Work out the finished part from the listing and answer in its coordinate system (mm). A direction names the side the tool comes from. Round coordinates to 2 decimals unless told otherwise and drop trailing zeros. Loops run counter-clockwise (first coordinate to the right, second up) from the corner with the lowest first, then second, coordinate; pieces in that order, holes last.
```python
from build123d import *

# Parameters (mm, degrees)
F1_DEPTH = 1000


with BuildPart() as f1:
    # F0 (on Right) → F1 (new body)
    with BuildSketch(Plane.YZ):
        with BuildLine():
            Line((0, 73.95), (0, 0.5))
            ThreePointArc((0, 0.5), (0.146447, 0.146447), (0.5, 0))
            Line((0.5, 0), (1.1, 0))
            ThreePointArc((1.1, 0), (1.453553, 0.146447), (1.6, 0.5))
            Line((1.6, 0.5), (1.6, 76.2))
            Line((1.6, 76.2), (77.798804, 76.2))
            Line((77.798804, 76.2), (77.798804, 77.2))
            Line((77.798804, 77.2), (1.598804, 77.2))
            Line((1.598804, 77.2), (1.598804, 79.3))
            Line((1.598804, 79.3), (2.548804, 79.3))
            ThreePointArc((2.548804, 79.3), (2.696007, 79.118338), (2.919614, 79.05))
            Line((2.919614, 79.05), (3.348827, 79.05))
            ThreePointArc((3.348827, 79.05), (3.524228, 79.121858), (3.598797, 79.296124))
            Line((3.598797, 79.296124), (3.598857, 79.3))
            Line((3.598857, 79.3), (3.598857, 80.9))
            Line((3.598857, 80.9), (0, 80.9))
            Line((0, 80.9), (0, 75.55))
            Line((0, 75.55), (-1.85, 75.55))
            Line((-1.85, 75.55), (-1.85, 73.95))
            ThreePointArc((-1.85, 73.95), (-1.776777, 73.773223), (-1.6, 73.7))
            Line((-1.6, 73.7), (-1.22081, 73.7))
            ThreePointArc((-1.22081, 73.7), (-0.997203, 73.768338), (-0.85, 73.95))
            Line((-0.85, 73.95), (0, 73.95))
        make_face()
    extrude(amount=F1_DEPTH)


solid = f1.part
```
1. Given pin 1 (2 mm diameter, centred on x = 269.5, z = 64, fed in from -Y); pin 2 (0.6 mm diameter, centred on x = 342, y = -0.5, fed in from +Z); pin 3 (12 mm diameter, centred on x = 673, y = 61, fed in from -Z), each flat-ended and moving along its own axis, determine where each tip first touches the part or whether it passes through.
Answer key:
pin 1: stops at y = 0
pin 2: stops at z = 75.55
pin 3: stops at z = 76.2
2. Which of the six approach directions +Z, -Z, +X, -X, +Y, -Y give full straight-line access (tool end or side, diameter ignored) to faces 1 (the face through (1000, 38, 77)), 2 (the face through (493, 0, 38)), 3 (the face through (493, 1.6, 38))?
Answer key:
face 1: +Z, -Z, +X, +Y, -Y
face 2: -Z, +X, -X, -Y
face 3: -Z, +X, -X, +Y
3. Find section B-B (y = 52.5). Write down the section's boundary in (x, z), then the cut area to 3 significant figures.
Answer key:
outline: (0, 76.2) - (1000, 76.2) - (1000, 77.2) - (0, 77.2) - close
area: 1,000 mm2
4. Find section C-C (z = 38). Write down the section's boundary in (x, y), then the cut area to 3 significant figures.
Answer key:
outline: (0, 0) - (1000, 0) - (1000, 1.6) - (0, 1.6) - close
area: 1,600 mm2
5. Consider probe 1 along Z at (x, y) = (707, 7.5); probe 2 along Y at (x, z) = (280.5, 75); probe 3 along Y at (x, z) = (841, 25.5). Determine where each line is inside the solid, lowest interval first.
Answer key:
probe 1: z = 76.2 to 77.2
probe 2: y = -1.85 to 1.6
probe 3: y = 0 to 1.6
